Print and shaded views of the part. All mm, measured from the part's lowest x, y and z. Coordinates: 2 decimals unless noted, no trailing zeros. Loops run counter-clockwise (first coordinate to the right, second up) from the corner with the lowest first, then second, coordinate; pieces in that order, holes last.
1) Saw through at C-C, the plane z = 38. Write the cut outline in (x, y), and give its area (3 significant figures).
2) Saw through at A-A, the plane x = 10.25. Write the cut outline in (y, z).
3) Wall check: line 1 along Z through (x, y) = (12, 298); line 2 along Y through (x, z) = (6.75, 39.5); line 3 along X through (y, z) = (69, 54.5). Give the ranges that are in metal, low to high.
4) Pin check, flat tips, straight feed: pin 1 Ø1.9 at (x, y) = (9.5, 223.5) entering from -Z; pin 2 Ø1 at (y, z) = (316, 53.5) entering from +X; pin 3 Ø7 at (x, z) = (11, 4.5) entering from -Y; pin 4 Ø5 at (x, z) = (11, 3) entering from +Y. Stop position of each tip, or through.
5) Saw through at B-B, the plane y = 43. Write the cut outline in (x, z).
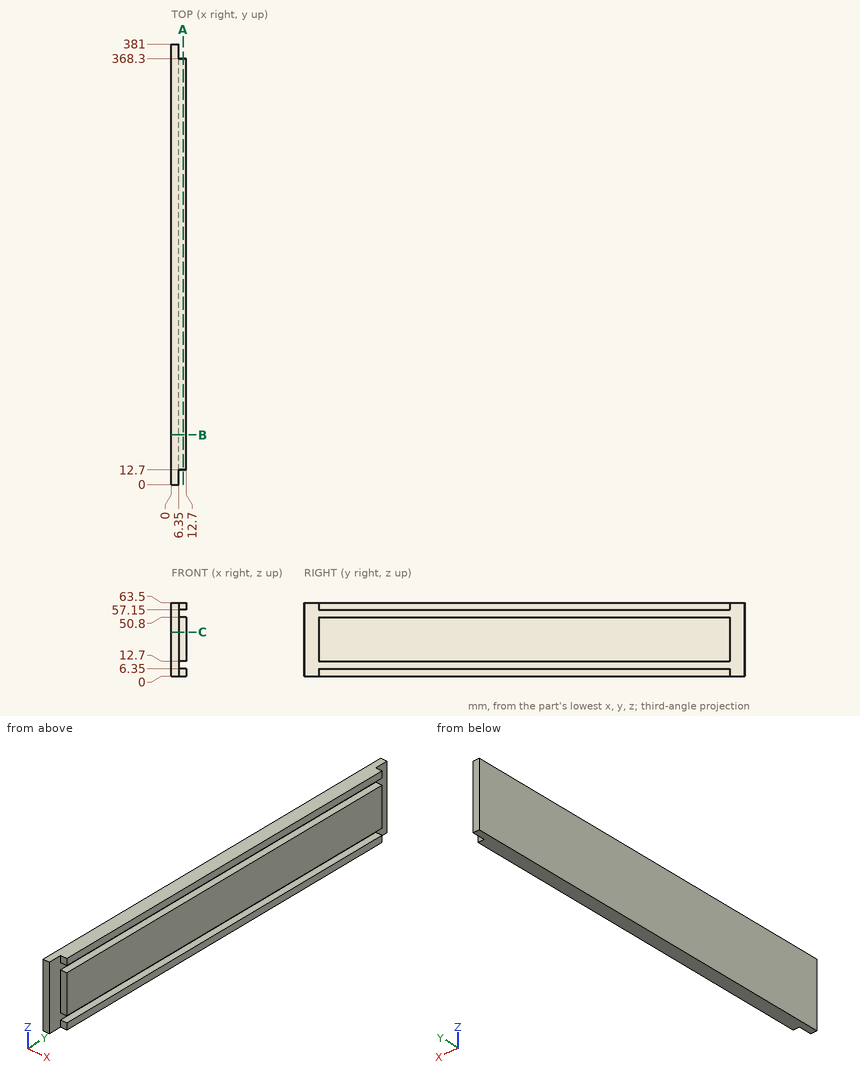
Data:
1. outline: (0, 0) - (6.35, 0) - (6.35, 12.7) - (12.7, 12.7) - (12.7, 368.3) - (6.35, 368.3) - (6.35, 381) - (0, 381) - close
1. area: 4,680 mm2
2. outline: (12.7, 0) - (368.3, 0) - (368.3, 6.35) - (12.7, 6.35) - close; (12.7, 12.7) - (368.3, 12.7) - (368.3, 50.8) - (12.7, 50.8) - close; (12.7, 57.15) - (368.3, 57.15) - (368.3, 63.5) - (12.7, 63.5) - close
3. line 1: z = 0 to 6.35, 12.7 to 50.8, 57.15 to 63.5
3. line 2: y = 12.7 to 368.3
3. line 3: x = 0 to 6.35
4. pin 1: stops at z = 0
4. pin 2: stops at x = 6.35
4. pin 3: stops at y = 12.7
4. pin 4: stops at y = 368.3
5. outline: (0, 0) - (12.7, 0) - (12.7, 6.35) - (6.35, 6.35) - (6.35, 12.7) - (12.7, 12.7) - (12.7, 50.8) - (6.35, 50.8) - (6.35, 57.15) - (12.7, 57.15) - (12.7, 63.5) - (0, 63.5) - close
